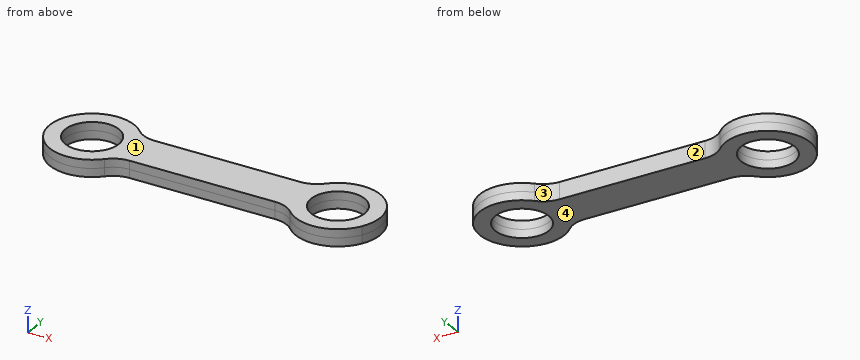
from build123d import *

# Parameters (mm, degrees)
SZKIC1_R                    = 9.5
DODANIE_WYCI_GNI_CIE1_DEPTH = 3
ZAOKR_GLENIE1_R             = 10


with BuildPart() as part:
    # Szkic1 → Dodanie-wyciągnięcie1 (new, symmetric)
    with BuildSketch(Plane.XY):
        with BuildLine():
            Line((-12.990381057, 7.5), (-74.509618943, 7.5))
            ThreePointArc((-74.509618943, 7.5), (-94.991658931, 12.995193206), (-100.5, -7.483314774))
            ThreePointArc((-100.5, -7.483314774), (-87.509629653, -14.999996909), (-74.509618943, -7.5))
            Line((-74.509618943, -7.5), (-12.990381057, -7.5))
            ThreePointArc((-12.990381057, -7.5), (0, -15), (12.990381057, -7.5))
            ThreePointArc((12.990381057, -7.5), (7.5, 12.990381057), (-12.990381057, 7.5))
        make_face()
        with Locations((-87.5, 0)):
            Circle(SZKIC1_R, mode=Mode.SUBTRACT)
        Circle(SZKIC1_R, mode=Mode.SUBTRACT)
    extrude(amount=DODANIE_WYCI_GNI_CIE1_DEPTH, both=True)

    # Zaokrąglenie1
    zaokr_glenie1_edges = [part.edges().sort_by_distance(p)[0] for p in [
        (-74.509618943, 7.5, -1.5),
        (-12.990381057, 7.5, -1.5),
        (-12.990381057, -7.5, -1.5),
        (-74.509618943, -7.5, -1.5),
    ]]
    fillet(zaokr_glenie1_edges, radius=ZAOKR_GLENIE1_R)


solid = part.part
Source: CAD feature listing. Evaluate the final solid. Frame: model axes, mm. Face numbers are marked on the shaded views. A direction names the side the tool comes from. Give positions to 0.01 mm unless a question says otherwise; leave off trailing zeros. Write each loop counter-clockwise with the first axis right and the second up, starting at its lowest first coordinate (ties: lowest second). Pieces come first, ordered by that corner, then holes. Notation, with made-up numbers: (42.5, 12) - (79.5, 12) arc R6 cw to (79.5, 23) - close; hole circle Ø9 at (-4, -7.75). An arc over 180 degrees is marked (long way). Write item = value, one per line. Start each with the question number.
Q1. Draft query along X for the marked faces 3 and 4. Return one class per face: +X half, -X half, draft (parallel to the pull), parting line (faces both ways), or undercut.
Q2. Reachability of the marked faces 1 and 2 from +Z, -Z, +X, -X, +Y, -Y: full face, straight path, thin tool, end or side. Return the list, or none.
Q3. Cut plane A-A, the plane x = -87.5. Return loops of the section in (y, z).
Q4. Material intervals for probe 1 along Y at (x, z) = (-87.5, 1); probe 2 along X at (y, z) = (7, 2.1); probe 3 along X at (y, z) = (-3.5, 1.5), sorted ascending.
Q5. Cut plane B-B, the plane z = -1. Return loops of the section in (x, y).
Q6. Pin query (flat end, axial travel): pin 1 Ø1.5 at (x, z) = (-74, 1) entering from +Y; pin 2 Ø0.9 at (x, z) = (-33, 1.5) entering from -Y; pin 3 Ø1.5 at (y, z) = (7, 0) entering from +X. Return the tip coordinate at first contact, or that it passes through.
Q7. Cut plane D-D, the plane y = -13. Return loops of the section in (x, z), then the cut area to 3 significant figures.
Q8. Cut plane C-C, the plane y = 0. Return loops of the section in (x, z).
Computed values:
q1.face_3 = undercut
q1.face_4 = draft
q2.face_1 = +Z, +X, -X, +Y, -Y
q2.face_2 = +Z, -Z, +Y
q3.outline = (-15, -3) - (-9.5, -3) - (-9.5, 3) - (-15, 3) - close; (9.5, -3) - (15, -3) - (15, 3) - (9.5, 3) - close
q4.probe_1 = -15 to -9.5, 9.5 to 15
q4.probe_2 = -100.77 to -93.92, -81.08 to -6.42, 6.42 to 13.27
q4.probe_3 = -102.09 to -96.33, -78.67 to -8.83, 8.83 to 14.59
q5.outline = (-76.79, -10.5) arc R10 cw to (-69.65, -7.5) - (-17.85, -7.5) arc R10 cw to (-10.71, -10.5) arc R15 ccw (long way) to (-10.71, 10.5) arc R10 cw to (-17.85, 7.5) - (-69.65, 7.5) arc R10 cw to (-76.79, 10.5) arc R15 ccw (long way) to start; hole circle Ø19 at (-87.5, 0); hole circle Ø19 at (0, 0)
q6.pin_1 = 8.9
q6.pin_2 = -7.5
q6.pin_3 = 13.64
q7.outline = (-94.98, -3) - (-80.02, -3) - (-80.02, 3) - (-94.98, 3) - close; (-7.48, -3) - (7.48, -3) - (7.48, 3) - (-7.48, 3) - close
q7.area = 180 mm²
q8.outline = (-102.5, -3) - (-97, -3) - (-97, 3) - (-102.5, 3) - close; (-78, -3) - (-9.5, -3) - (-9.5, 3) - (-78, 3) - close; (9.5, -3) - (15, -3) - (15, 3) - (9.5, 3) - close
